Here's how the part is built. I have some questions about the finished solid (model axes, mm). Face numbers are marked on the shaded views. A direction names the side the tool comes from. Round coordinates to 2 decimals unless told otherwise and drop trailing zeros. Write each loop counter-clockwise with the first axis right and the second up, starting at its lowest first coordinate (ties: lowest second). Pieces come first, ordered by that corner, then holes. Notation, with made-up numbers: (44, -2.75) - (58, -2.75) arc R6 cw to (58, 3.25) - close; hole circle Ø4 at (59.5, 75). An arc over 180 degrees is marked (long way). One line per item, written item: value. Start each with the question number.
Item 1: For P1, Ø12, axis at y = 11, z = -18, coming from the +X side; P2, Ø15, axis at y = 22, z = -12, coming from the -X side; P3, Ø3, axis at y = 21.5, z = -26.5, coming from the -X side, each with a flat end and sliding along its axis, tell me the tip position at first contact or that it passes through.
Item 2: Thinking about a two-plate mould opening in Z: for the marked faces 4, 5 and 6, which applies, released by +Z, released by -Z, zero draft, split by the parting line, or undercut?
Item 3: If I drill on line 1 (Z direction, x = 33, y = 52.45); line 2 (X direction, y = 51.7, z = -10); line 3 (Y direction, x = 27.5, z = -9), over which ranges is the centre line in solid material (lowest first)?
Item 4: For the marked faces 1, 2 and 3, which set-ups out of +Z, -Z, +X, -X, +Y, -Y let a thin tool reach every point of the face, with its end or its side?
Item 5: Imagine slicing it at D-D, the plane x = 24. Please give me the cut outline in (y, z), then the cut area to 3 significant figures.
Item 6: Imagine slicing it at B-B, the plane x = -5. Please give me the cut outline in (y, z), then the cut area to 3 significant figures.
Item 7: Imagine slicing it at A-A, the plane z = -10. Please give me the cut outline in (x, y) (3 decimals).
Item 8: Imagine slicing it at C-C, the plane y = 33. Please give me the cut outline in (x, z).
```python
from build123d import *

# Parameters (mm, degrees)
BOSS_EXTRUDE1_DEPTH            = 55
BOSS_EXTRUDE2_START            = 55
BOSS_EXTRUDE2_DEPTH            = 5
M3_CLEARANCE_HOLE1_D           = 3.4
M3_CLEARANCE_HOLE1_CSINK_D     = 3.45
M3_CLEARANCE_HOLE1_CSINK_ANGLE = 90


with BuildPart() as part:
    # Sketch1 → Boss-Extrude1 (new body)
    with BuildSketch(Plane(origin=(0, 0, 0), x_dir=(1, 0, 0), z_dir=(0, 1, 0))):
        Polygon((3, 0), (0, 0), (0, 18.87138772), (-13.505514799, 34.280690781), (-13.505514799, 57.637057616), (7.616499063, 78.521745479), (7.592529724, 74.279172502), (-10.505514799, 56.384476794), (-10.505514799, 35.409303061), (3, 20), align=None)
    extrude(amount=BOSS_EXTRUDE1_DEPTH)

    # Sketch1<3> → Boss-Extrude2 (add)
    with BuildSketch(Plane(origin=(0, 0, 0), x_dir=(1, 0, 0), z_dir=(0, 1, 0)).offset(BOSS_EXTRUDE2_START)):
        with BuildLine():
            Line((3, 17.5), (3, 2.5))
            Line((3, 2.5), (33, 2.5))
            ThreePointArc((33, 2.5), (40.5, 10), (33, 17.5))
            Line((33, 17.5), (3, 17.5))
        make_face()
    extrude(amount=-BOSS_EXTRUDE2_DEPTH)

    # M3 Clearance Hole1 (through all)
    with Locations(Plane(origin=(0, 55, 0), x_dir=(1, 0, 0), z_dir=(0, 1, 0))):
        with Locations((33, 10)):
            CounterSinkHole(M3_CLEARANCE_HOLE1_D / 2, M3_CLEARANCE_HOLE1_CSINK_D / 2, counter_sink_angle=M3_CLEARANCE_HOLE1_CSINK_ANGLE)


solid = part.part
```
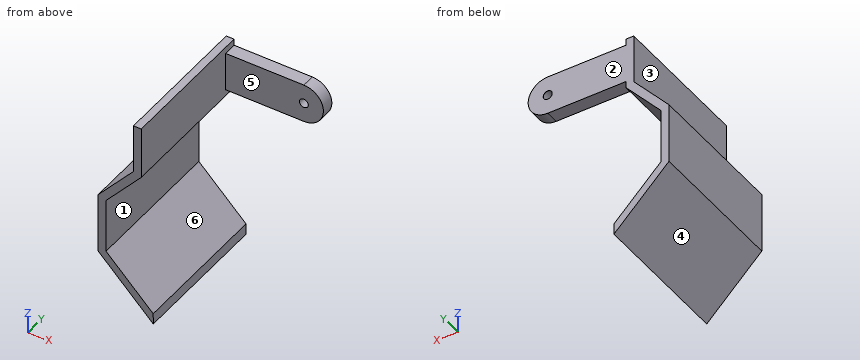
Values follow:
1. P1: stops at x = 3
1. P2: stops at x = -0.55
1. P3: stops at x = -8
2. face 4: released by -Z
2. face 5: zero draft
2. face 6: undercut
3. line 1: z = -17.5 to -11.7, -8.3 to -2.5
3. line 2: x = 0 to 31.3, 34.7 to 40.5
3. line 3: y = 50 to 55
4. face 1: +X, +Y, -Y
4. face 2: +Z, -Z, +X, -X, +Y
4. face 3: +Z, -X, +Y, -Y
5. outline: (50, -17.5) - (55, -17.5) - (55, -2.5) - (50, -2.5) - close
5. area: 75.0 mm^2
6. outline: (0, -66.05) - (55, -66.05) - (55, -61.83) - (0, -61.83) - close; (0, -29.13) - (55, -29.13) - (55, -24.58) - (0, -24.58) - close
6. area: 482 mm^2
7. outline: (0, 0) - (3, 0) - (3, 50) - (31.3, 50) - (31.3, 54.975) - (31.275, 55) - (0, 55) - close; (34.7, 50) - (40.5, 50) - (40.5, 55) - (34.725, 55) - (34.7, 54.975) - close
8. outline: (-13.51, -57.64) - (7.62, -78.52) - (7.59, -74.28) - (-10.51, -56.38) - (-10.51, -35.41) - (3, -20) - (3, 0) - (0, 0) - (0, -18.87) - (-13.51, -34.28) - close
